Verification items for the finished model (mm, model axes). Coordinates: 2 decimals unless noted, no trailing zeros. Write each loop counter-clockwise with the first axis right and the second up, starting at its lowest first coordinate (ties: lowest second). Pieces come first, ordered by that corner, then holes. Notation, with made-up numbers: (66.25, 4) -> (76.25, 4) arc R24 cw to (76.25, 14) -> close; hole circle Ø5 at (21, -4). An arc over 180 degrees is marked (long way). Answer in a Markdown table with one row per item.
Autodesk Inventor part; units mm, degrees
ref_plane "YZ Plane" through (0, 0, 0) normal (1, 0, 0) x (0, 1, 0)
ref_plane "XZ Plane" through (0, 0, 0) normal (0, 1, 0) x (-1, 0, 0)
ref_plane "XY Plane" through (0, 0, 0) normal (0, 0, 1) x (1, 0, 0)
sketch "Sketch1" plane through (0, 0, 0) normal (0, 0, 1) x (1, 0, 0)
  line L0 (0, 35.7) -> (0, -35.7) construction
  line L1 (-63, 0) -> (63, 0) construction
  line L2 (45, -25.5) -> (-45, -25.5)
  line L3 (-45, -25.5) -> (-45, 25.5)
  line L4 (-45, 25.5) -> (45, 25.5)
  line L5 (45, 25.5) -> (45, -25.5)
  line L6 (45, -25.5) -> (-45, 25.5) construction
  line L7 (-45, -25.5) -> (45, 25.5) construction
  point P0 (0, 0)
  dimension "d0" = 90
  dimension "d1" = 51
extrude "Extrusion1" add sketch "Sketch1" along normal mid plane 0.8
sketch "Esquisse2" plane through (0, 0, 0.4) normal (0, 0, 1) x (1, 0, 0)
  line L0 (-45, -25.5) -> (45, -25.5) construction
  line L1 (45, -25.5) -> (45, 25.5) construction
  line L2 (45, 25.5) -> (-45, 25.5) construction
  line L3 (-45, 25.5) -> (-45, -25.5) construction
  line L4 (-63, 0) -> (63, 0) construction
  line L5 (0, 35.7) -> (0, -35.7) construction
  circle A0 centre (-13, -15) radius 9
  circle A1 centre (13, -15) radius 9
  point P0 (0, 0)
  dimension "d4" = 10.5
  dimension "d5" = 18
  dimension "d6" = 18
  dimension "d7" = 26
extrude "Extrusion2" cut sketch "Esquisse2" against normal through all
sketch "Esquisse3" plane through (0, 0, 0.4) normal (0, 0, 1) x (1, 0, 0)
  circle A0 centre (-13, -15) radius 9 construction
  circle A1 centre (13, -15) radius 9 construction
  line L0 (-45, -25.5) -> (45, -25.5) construction
  line L1 (45, -25.5) -> (45, 25.5) construction
  line L2 (45, 25.5) -> (-45, 25.5) construction
  line L3 (-45, 25.5) -> (-45, -25.5) construction
  line L4 (-63, 0) -> (63, 0) construction
  line L5 (0, 35.7) -> (0, -35.7) construction
  line L6 (-5.75, -21) -> (5.75, -21)
  line L7 (5.75, -21) -> (5.75, -25.5)
  line L8 (5.75, -25.5) -> (-5.75, -25.5)
  line L9 (-5.75, -25.5) -> (-5.75, -21)
  point P0 (0, 0)
  dimension "d10" = 4.5
  dimension "d11" = 11.5
extrude "Extrusion3" cut sketch "Esquisse3" against normal through all
sketch "Esquisse4" plane through (0, 0, 0.4) normal (0, 0, 1) x (1, 0, 0)
  line L0 (5.75, -21) -> (5.75, -25.5) construction
  line L1 (5.75, -25.5) -> (45, -25.5) construction
  line L2 (45, -25.5) -> (45, 25.5) construction
  line L3 (45, 25.5) -> (-45, 25.5) construction
  line L4 (-45, 25.5) -> (-45, -25.5) construction
  line L5 (-45, -25.5) -> (-5.75, -25.5) construction
  line L6 (-5.75, -25.5) -> (-5.75, -21) construction
  line L7 (-5.75, -21) -> (5.75, -21) construction
  circle A0 centre (-13, -15) radius 9 construction
  circle A1 centre (13, -15) radius 9 construction
  line L8 (0, 35.7) -> (0, -35.7) construction
  line L9 (-63, 0) -> (63, 0) construction
  line L10 (-38, 21.5) -> (38, 21.5)
  line L11 (38, 21.5) -> (38, -1.5)
  line L12 (38, -1.5) -> (-38, -1.5)
  line L13 (-38, -1.5) -> (-38, 21.5)
  point P0 (0, 0)
  dimension "d14" = 76
  dimension "d15" = 23
  dimension "d16" = 4
extrude "Extrusion4" cut sketch "Esquisse4" against normal blind 10
sketch "Esquisse5" plane through (0, 0, 0.4) normal (0, 0, 1) x (1, 0, 0)
  line L0 (-38, -1.5) -> (-38, 21.5) construction
  line L1 (-38, 21.5) -> (38, 21.5) construction
  line L2 (38, 21.5) -> (38, -1.5) construction
  line L3 (38, -1.5) -> (-38, -1.5) construction
  line L4 (5.75, -21) -> (5.75, -25.5) construction
  line L5 (5.75, -25.5) -> (45, -25.5) construction
  line L6 (45, -25.5) -> (45, 25.5) construction
  line L7 (45, 25.5) -> (-45, 25.5) construction
  line L8 (-45, 25.5) -> (-45, -25.5) construction
  line L9 (-45, -25.5) -> (-5.75, -25.5) construction
  line L10 (-5.75, -25.5) -> (-5.75, -21) construction
  line L11 (-5.75, -21) -> (5.75, -21) construction
  circle A0 centre (-13, -15) radius 9 construction
  circle A1 centre (13, -15) radius 9 construction
  line L12 (-41, -11.5) -> (-27, -11.5)
  line L13 (-27, -11.5) -> (-27, -21.5)
  line L14 (-27, -21.5) -> (-41, -21.5)
  line L15 (-41, -21.5) -> (-41, -11.5)
  line L16 (0, 35.7) -> (0, -35.7) construction
  line L17 (41, -11.5) -> (27, -11.5)
  line L18 (27, -11.5) -> (27, -21.5)
  line L19 (27, -21.5) -> (41, -21.5)
  line L20 (41, -21.5) -> (41, -11.5)
  point P0 (0, 0)
  dimension "d19" = 14
  dimension "d20" = 10
  dimension "d21" = 4
  dimension "d22" = 4
extrude "Extrusion5" cut sketch "Esquisse5" against normal blind 10
sketch "Esquisse7" plane through (0, 0, -0.4) normal (0, 0, -1) x (-1, 0, 0)
  line L0 (44.2, 0.8021) -> (45, 0.8021)
  line L1 (45, 0.8021) -> (45, -7.1979)
  line L2 (45, -7.1979) -> (44.2, -7.1979)
  line L3 (44.2, -7.1979) -> (44.2, 0.8021)
  line L4 (44.2, 15.8021) -> (45, 15.8021)
  line L5 (45, 15.8021) -> (45, 7.8021)
  line L6 (45, 7.8021) -> (44.2, 7.8021)
  line L7 (44.2, 7.8021) -> (44.2, 15.8021)
  line L8 (44.2, -14.1979) -> (45, -14.1979)
  line L9 (45, -14.1979) -> (45, -22.1979)
  line L10 (45, -22.1979) -> (44.2, -22.1979)
  line L11 (44.2, -22.1979) -> (44.2, -14.1979)
  line L12 (-45, 0.8021) -> (-44.2, 0.8021)
  line L13 (-44.2, 0.8021) -> (-44.2, -7.1979)
  line L14 (-44.2, -7.1979) -> (-45, -7.1979)
  line L15 (-45, -7.1979) -> (-45, 0.8021)
  line L16 (-45, 15.8021) -> (-44.2, 15.8021)
  line L17 (-44.2, 15.8021) -> (-44.2, 7.8021)
  line L18 (-44.2, 7.8021) -> (-45, 7.8021)
  line L19 (-45, 7.8021) -> (-45, 15.8021)
  line L20 (-45, -14.1979) -> (-44.2, -14.1979)
  line L21 (-44.2, -14.1979) -> (-44.2, -22.1979)
  line L22 (-44.2, -22.1979) -> (-45, -22.1979)
  line L23 (-45, -22.1979) -> (-45, -14.1979)
  point P0 (0, 0)
extrude "Extrusion7" cut sketch "Esquisse7" against normal blind 0.8
properties part number "Carosserie_Capot_Avant_Bas" material "PVC-U"
1. Sectioned sample at C-C, the plane x = -25.5. Record the cut outline in (y, z).
Findings below:
| item | result |
|---|---|
| outline | (-25.5, -0.4) -> (-1.5, -0.4) -> (-1.5, 0.4) -> (-25.5, 0.4) -> close; (21.5, -0.4) -> (25.5, -0.4) -> (25.5, 0.4) -> (21.5, 0.4) -> close |
2. Sectioned sample at A-A, the plane x = -13. Record the cut outline in (y, z), and give its area (3 significant figures).
Findings below:
| item | result |
|---|---|
| outline | (-25.5, -0.4) -> (-24, -0.4) -> (-24, 0.4) -> (-25.5, 0.4) -> close; (-6, -0.4) -> (-1.5, -0.4) -> (-1.5, 0.4) -> (-6, 0.4) -> close; (21.5, -0.4) -> (25.5, -0.4) -> (25.5, 0.4) -> (21.5, 0.4) -> close |
| area | 8.00 mm² |
3. Material ranges on probe 1 along Y at (x, z) = (13, 0.3); probe 2 along Y at (x, z) = (31.5, 0.2); probe 3 along X at (y, z) = (10, 0.3), recorded low to high. Write a range as from..to.
Findings below:
| item | result |
|---|---|
| probe 1 | y = -25.5..-24, -6..-1.5, 21.5..25.5 |
| probe 2 | y = -25.5..-21.5, -11.5..-1.5, 21.5..25.5 |
| probe 3 | x = -44.2..-38, 38..44.2 |
4. Release check for a two-part mould opening along Y. For faces 1 (the face through (-8.847, -22.985, 0.006)), 2 (the face through (-1, -5, -0.4)) record: released by +Y, released by -Y, zero draft, split by the parting line, or undercut.
Findings below:
| item | result |
|---|---|
| face 1 | undercut |
| face 2 | zero draft |
5. Go/stop test with a flat-tipped pin: pin 1 (3 mm diameter, centred on x = 20.5, y = -12.5, fed in from -Z). Record where the tip stops, or that it passes through.
Findings below:
| item | result |
|---|---|
| pin 1 | stops at z = -0.4 |
6. Sectioned sample at D-D, the plane z = 0.1. Count the separate pieces of the cut face and the enclosed holes in it, and give its area (3 significant figures).
Findings below:
| item | result |
|---|---|
| separate pieces | 1 |
| enclosed holes | 5 |
| area | 1,960 mm² |
7. Sectioned sample at B-B, the plane y = 4. Record the cut outline in (x, z).
Findings below:
| item | result |
|---|---|
| outline | (-45, -0.4) -> (-38, -0.4) -> (-38, 0.4) -> (-45, 0.4) -> close; (38, -0.4) -> (45, -0.4) -> (45, 0.4) -> (38, 0.4) -> close |
